from build123d import *

# Parameters (mm, degrees)
SKETCH1_W           = 40
SKETCH1_H           = 40
BOSS_EXTRUDE1_DEPTH = 40
CUT_EXTRUDE1_DEPTH  = 20


with BuildPart() as part:
    # Sketch1 → Boss-Extrude1 (new body)
    with BuildSketch(Plane.XY):
        with Locations((20, 20)):
            Rectangle(SKETCH1_W, SKETCH1_H)
    extrude(amount=BOSS_EXTRUDE1_DEPTH)

    # Sketch2 → Cut-Extrude1 (cut)
    with BuildSketch(Plane(origin=(0, 40, 0), x_dir=(1, 0, 0), z_dir=(0, 1, 0))):
        Polygon((0, 0), (40, -40), (40, 0), align=None)
    extrude(amount=-CUT_EXTRUDE1_DEPTH, mode=Mode.SUBTRACT)


solid = part.part
Can you work these out from the model? Positions are in its coordinate system, mm. A direction names the side the tool comes from. Coordinates: 2 decimals unless noted, no trailing zeros. Loops run counter-clockwise (first coordinate to the right, second up) from the corner with the lowest first, then second, coordinate; pieces in that order, holes last. Notation, with made-up numbers: (76.5, 28) - (130.5, 28) arc R12 cw to (130.5, 38) - close; hole circle Ø2 at (-17.5, 18.25). An arc over 180 degrees is marked (long way). Put each result on its own line as item: value. Start each with the question number.
Item 1: Suppose I cut it at A-A (x = 14). Please give me the cut outline in (y, z).
Item 2: Which directions (+Z, -Z, +X, -X, +Y, -Y) give clear straight access to the entire face, cutting with the end or side of a thin tool? Please do faces 1 (the face through (20, 30, 20)), 2 (the face through (40, 10, 20)).
Item 3: Suppose I cut it at B-B (z = 14.5). Please give me the cut outline in (x, y), and give its area (3 significant figures).
Item 4: Suppose I cut it at C-C (y = 34.5). Please give me the cut outline in (x, z).
Item 5: For pin 1 (6 mm diameter, centred on x = 11, z = 13.5, fed in from -Y); pin 2 (3 mm diameter, centred on x = 24.5, z = 10, fed in from +Y), each with a flat end and sliding along its axis, tell me the tip position at first contact or that it passes through.
Item 6: If I drill on line 1 along Y through (x, z) = (35, 27); line 2 along Z through (x, y) = (25, 20.5); line 3 along X through (y, z) = (30.5, 27), over which ranges is the centre line in solid material (lowest first)?
Here are the results:
1. outline: (0, 0) - (20, 0) - (20, 14) - (40, 14) - (40, 40) - (0, 40) - close
2. face 1: -Z, +X, +Y
2. face 2: +Z, -Z, +X, +Y, -Y
3. outline: (0, 0) - (40, 0) - (40, 20) - (14.5, 20) - (14.5, 40) - (0, 40) - close
3. area: 1,090 mm²
4. outline: (0, 0) - (40, 40) - (0, 40) - close
5. pin 1: y = 0
5. pin 2: y = 20
6. line 1: 0 to 20
6. line 2: 25 to 40
6. line 3: 0 to 27
